Could you check a few things on this model? Use its own coordinates, in mm. A direction names the side the tool comes from. Round coordinates to 2 decimals unless told otherwise and drop trailing zeros. Write each loop counter-clockwise with the first axis right and the second up, starting at its lowest first coordinate (ties: lowest second). Pieces come first, ordered by that corner, then holes. Notation, with made-up numbers: (8, 1) - (31, 1) arc R28 ccw to (31, 35) - close; hole circle Ø5 at (-36, -7.5). An arc over 180 degrees is marked (long way). Put each result on its own line as item: value.
from build123d import *

# Parameters (mm, degrees)
SKETCH1_W                                            = 25
SKETCH1_H                                            = 37
BOSS_EXTRUDE2_DEPTH                                  = 20
SKETCH4_W                                            = 23.2
SKETCH4_H                                            = 35.3
CUT_EXTRUDE1_DEPTH                                   = 18
SKETCH30_W                                           = 10
SKETCH30_H                                           = 10
BOSS_EXTRUDE5_DEPTH                                  = 3
CBORE_FOR_M3_HEXAGON_HEAD_BOLTS_FULL_THR_D           = 3.4
CBORE_FOR_M3_HEXAGON_HEAD_BOLTS_FULL_THR_CBORE_D     = 9
CBORE_FOR_M3_HEXAGON_HEAD_BOLTS_FULL_THR_CBORE_DEPTH = 0.5
SKETCH32_W                                           = 25
SKETCH32_H                                           = 37
CUT_EXTRUDE2_DEPTH                                   = 5


with BuildPart() as part:
    # Sketch1 → Boss-Extrude2 (new body)
    with BuildSketch(Plane(origin=(0, 0, 0), x_dir=(1, 0, 0), z_dir=(0, 1, 0))):
        with Locations((-76.226170177, 10.94482429)):
            Rectangle(SKETCH1_W, SKETCH1_H)
    extrude(amount=BOSS_EXTRUDE2_DEPTH)

    # Sketch4 → Cut-Extrude1 (cut)
    with BuildSketch(Plane(origin=(0, 20, 0), x_dir=(1, 0, 0), z_dir=(0, 1, 0))):
        with Locations((-76.226170177, 10.94482429)):
            Rectangle(SKETCH4_W, SKETCH4_H)
    extrude(amount=-CUT_EXTRUDE1_DEPTH, mode=Mode.SUBTRACT)

    # Sketch30 → Boss-Extrude5 (add)
    with BuildSketch(Plane.ZY.offset(88.726170177)):
        with Locations((-34.44482429, 10)):
            Rectangle(SKETCH30_W, SKETCH30_H)
        with Locations((12.55517571, 10)):
            Rectangle(SKETCH30_W, SKETCH30_H)
    extrude(amount=-BOSS_EXTRUDE5_DEPTH)

    # CBORE for M3 Hexagon head bolts-Full thread-grades AB5 (through all)
    with Locations(Plane(origin=(-85.726170177, 10, -34.44482429), x_dir=(0, 0, 1), z_dir=(1, 0, 0))):
        with Locations((0, 0), (47, 0)):
            CounterBoreHole(CBORE_FOR_M3_HEXAGON_HEAD_BOLTS_FULL_THR_D / 2, CBORE_FOR_M3_HEXAGON_HEAD_BOLTS_FULL_THR_CBORE_D / 2, CBORE_FOR_M3_HEXAGON_HEAD_BOLTS_FULL_THR_CBORE_DEPTH)

    # Sketch32 → Cut-Extrude2 (cut)
    with BuildSketch(Plane.XZ):
        with Locations((-76.226170177, -10.94482429)):
            Rectangle(SKETCH32_W, SKETCH32_H)
    extrude(amount=-CUT_EXTRUDE2_DEPTH, mode=Mode.SUBTRACT)


solid = part.part
(1) I'm going to push flat-ended pins straight in: pin 1 (4.5 mm diameter, centred on x = -74.5, y = 10.5, fed in from -Z); pin 2 (8 mm diameter, centred on y = 11.5, z = -35.5, fed in from +X); pin 3 (4 mm diameter, centred on y = 10, z = 12.56, fed in from +X). Where does each tip first touch, or does it pass through?
Values found:
pin 1: stops at z = -29.44
pin 2: stops at x = -85.73
pin 3: stops at x = -86.23
(2) Imagine slicing it at C-C, the plane z = -24. List the corners of the cut face in (x, y) for me.
Values found:
outline: (-88.73, 5) - (-87.83, 5) - (-87.83, 20) - (-88.73, 20) - close; (-64.63, 5) - (-63.73, 5) - (-63.73, 20) - (-64.63, 20) - close
(3) Imagine slicing it at A-A, the plane y = 10. List the corners of the cut face in (x, z) for me.
Values found:
outline: (-88.73, -39.44) - (-85.73, -39.44) - (-85.73, -38.94) - (-86.23, -38.94) - (-86.23, -36.14) - (-88.73, -36.14) - close; (-88.73, -32.74) - (-86.23, -32.74) - (-86.23, -29.94) - (-85.73, -29.94) - (-85.73, -29.44) - (-63.73, -29.44) - (-63.73, 7.56) - (-85.73, 7.56) - (-85.73, 8.06) - (-86.23, 8.06) - (-86.23, 10.86) - (-88.73, 10.86) - close; (-88.73, 14.26) - (-86.23, 14.26) - (-86.23, 17.06) - (-85.73, 17.06) - (-85.73, 17.56) - (-88.73, 17.56) - close; hole (-87.83, -28.59) - (-64.63, -28.59) - (-64.63, 6.71) - (-87.83, 6.71) - close
(4) Imagine slicing it at B-B, the plane x = -74. List the corners of the cut face in (y, z) for me, then the cut area to 3 significant figures.
Values found:
outline: (5, -29.44) - (20, -29.44) - (20, -28.59) - (5, -28.59) - close; (5, 6.71) - (20, 6.71) - (20, 7.56) - (5, 7.56) - close
area: 25.5 mm^2
(5) For faces 4 (the face through (-87, 15, -35)), 5 (the face through (-87.826, 13, -11)), 6 (the face through (-87, 15, 12)), 7 (the face through (-85.726, 11, 8)), 8 (the face through (-85.973, 8.648, -30.153)), which set-ups out of +Z, -Z, +X, -X, +Y, -Y let a thin tool reach every point of the face, with its end or its side?
Values found:
face 4: -Z, +X, -X, +Y
face 5: +Y, -Y
face 6: +Z, +X, -X, +Y
face 7: +Z, +X, +Y, -Y
face 8: +X
(6) Imagine slicing it at D-D, the plane y = 7.5. List the corners of the cut face in (x, z) for me, then the cut area to 3 significant figures.
Values found:
outline: (-88.73, -39.44) - (-85.73, -39.44) - (-85.73, -38.19) - (-86.23, -38.19) - (-86.23, -30.7) - (-85.73, -30.7) - (-85.73, -29.44) - (-63.73, -29.44) - (-63.73, 7.56) - (-85.73, 7.56) - (-85.73, 8.81) - (-86.23, 8.81) - (-86.23, 16.3) - (-85.73, 16.3) - (-85.73, 17.56) - (-88.73, 17.56) - close; hole (-87.83, -28.59) - (-64.63, -28.59) - (-64.63, 6.71) - (-87.83, 6.71) - close
area: 159 mm^2
(7) Please list where these lines run through material, in increasing order: probe 1 along Z at (x, y) = (-87.1, 10); probe 2 along X at (y, z) = (15.25, -27.5); probe 3 along Z at (x, y) = (-84, 14). Write a range as from..to.
Values found:
probe 1: z = -39.44..-36.14, -32.74..-28.59, 6.71..10.86, 14.26..17.56
probe 2: x = -88.73..-87.83, -64.63..-63.73
probe 3: z = -29.44..-28.59, 6.71..7.56
(8) If we mould it in two halves opening along X, with no side actions, what happens to faces 1 (the face through (-86.226, 12, 12)), 2 (the face through (-76, 13, 6.705)), 3 (the face through (-87, 10, 17.555))? For each: pulls with the +X half, pulls with the -X half, needs draft (parallel to the pull), parting line crosses it, or undercut.
Values found:
face 1: pulls with the +X half
face 2: undercut
face 3: needs draft
